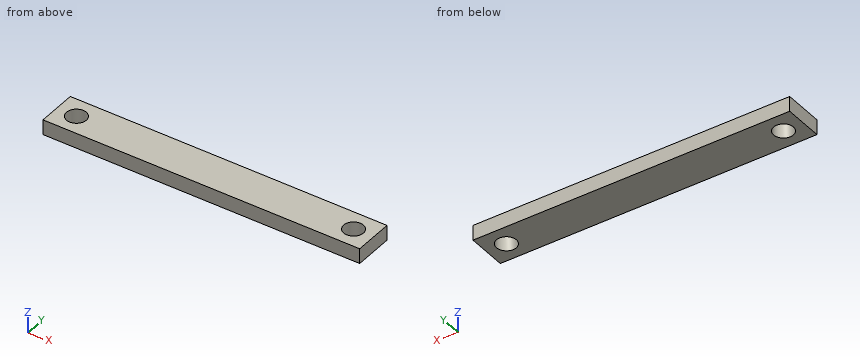
Autodesk Inventor part; units mm, degrees
ref_plane "YZ Plane" through (0, 0, 0) normal (1, 0, 0) x (0, 1, 0)
ref_plane "XZ Plane" through (0, 0, 0) normal (0, 1, 0) x (-1, 0, 0)
ref_plane "XY Plane" through (0, 0, 0) normal (0, 0, 1) x (1, 0, 0)
sketch "Sketch1" plane through (0, 0, 0) normal (0, 0, 1) x (1, 0, 0)
  line L0 (0, 0) -> (203.2, 0)
  line L1 (203.2, 0) -> (203.2, 25.4)
  line L2 (203.2, 25.4) -> (0, 25.4)
  line L3 (0, 25.4) -> (0, 0)
  circle A0 centre (12.7, 12.7) radius 6.35
  circle A1 centre (190.5, 12.7) radius 6.35
  dimension "d0" = 203.2
  dimension "d1" = 25.4
  dimension "d2" = 12.7
  dimension "d3" = 12.7
  dimension "d4" = 12.7
  dimension "d5" = 12.7
  dimension "d9" = 12.7
  dimension "d10" = 12.7
extrude "Extrusion1" add sketch "Sketch1" along normal blind 9.652
equation "\"d2\" = 0.5 * d1"
equation "\"d3\" = d2"
equation "\"d4\" = d2"
equation "\"d5\" = d3"
properties part number "GE-12024"
Input: part model. Units: mm. Frame: model coordinates. Give positions to 0.01 mm unless a question says otherwise; leave off trailing zeros. Write each loop counter-clockwise with the first axis right and the second up, starting at its lowest first coordinate (ties: lowest second). Pieces come first, ordered by that corner, then holes.
Q1. Section B-B, the plane x = 12.7. Output: boundary loops of the cut face in (y, z), plus the area to 3 significant figures.
Q2. Section A-A, the plane y = 12.7. Output: boundary loops of the cut face in (x, z).
Q3. Section C-C, the plane z = 2. Output: boundary loops of the cut face in (x, y).
Q4. Material intervals for probe 1 along Y at (x, z) = (12.7, 2.25); probe 2 along X at (y, z) = (16.25, 5.25); probe 3 along X at (y, z) = (8.75, 6.5), sorted ascending.
Filled in:
1. outline: (0, 0) - (6.35, 0) - (6.35, 9.65) - (0, 9.65) - close; (19.05, 0) - (25.4, 0) - (25.4, 9.65) - (19.05, 9.65) - close
1. area: 123 mm2
2. outline: (0, 0) - (6.35, 0) - (6.35, 9.65) - (0, 9.65) - close; (19.05, 0) - (184.15, 0) - (184.15, 9.65) - (19.05, 9.65) - close; (196.85, 0) - (203.2, 0) - (203.2, 9.65) - (196.85, 9.65) - close
3. outline: (0, 0) - (203.2, 0) - (203.2, 25.4) - (0, 25.4) - close; hole circle Ø12.7 at (12.7, 12.7); hole circle Ø12.7 at (190.5, 12.7)
4. probe 1: y = 0 to 6.35, 19.05 to 25.4
4. probe 2: x = 0 to 7.44, 17.96 to 185.24, 195.76 to 203.2
4. probe 3: x = 0 to 7.73, 17.67 to 185.53, 195.47 to 203.2
